Input: dimensioned drawing with shaded views. Units: mm. Origin: part minimum x, y, z. A direction names the side the tool comes from. Round coordinates to 2 decimals unless told otherwise and drop trailing zeros. Order: outer loops, then holes, each group sorted by start corner. A loop starts at its lowest first (then second) coordinate and runs counter-clockwise, first axis right, second up. Notation, with made-up numbers: (82.25, 55.25) - (89.25, 55.25) arc R24 cw to (89.25, 70.25) - close; hole circle Ø9 at (16.25, -10). An arc over 180 degrees is marked (long way). One line per item, written item: value. Start each with the question number.
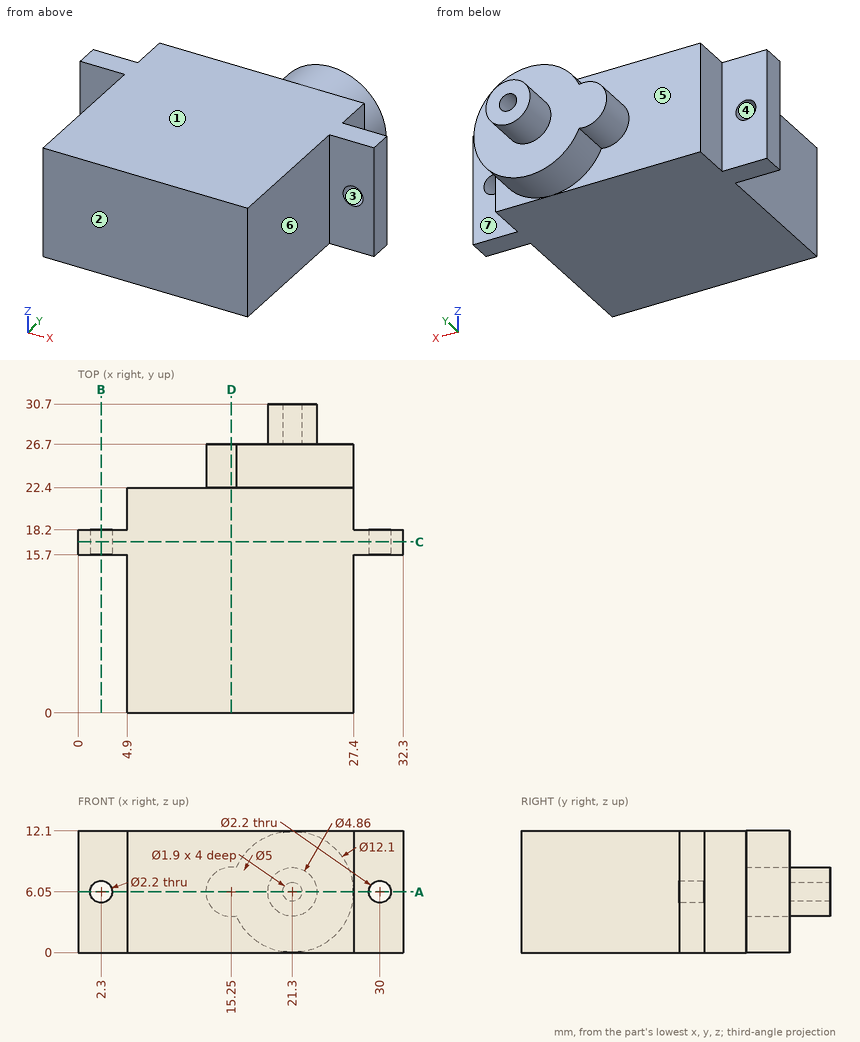
1. Set-up query: the marked faces 5, 6 and 7. Return all of +Z, -Z, +X, -X, +Y, -Y with unobstructed straight access to the full face (end or side cutting, diameter ignored); none if empty.
2. Section C-C (y = 17). Return the cut outline in (x, z).
3. Section A-A (z = 6.05). State how many separate pieces and enclosed holes the cut face has, then the cut area to 3 significant figures.
4. Section B-B (x = 2.3). Return the cut outline in (y, z), then the cut area to 4 significant figures.
5. Line query: line 1 (X direction, y = 16.7, z = 6.05); line 2 (X direction, y = 29.75, z = 6.05); line 3 (Z direction, x = 30, y = 17.2). Output: solid intervals per line, ascending. Write a range as from..to.
6. Pin query (flat end, axial travel): pin 1 (1.5 mm diameter, centred on x = 2.5, z = 7, fed in from -Y); pin 2 (8 mm diameter, centred on x = 18.5, y = 26, fed in from +Z); pin 3 (1.7 mm diameter, centred on x = 21.3, z = 6.05, fed in from +Y); pin 4 (6 mm diameter, centred on x = 11.5, y = 26, fed in from -Z). Return the tip coordinate at first contact, or that it passes through.
7. Section D-D (x = 15.25). Return the cut outline in (y, z), then the cut area to 3 significant figures.
8. Pull-direction query (Z, two-part tool) for the marked faces 1, 2, 3 and 4; classes: released by +Z, released by -Z, zero draft, split by the parting line, or undercut.
Solved:
1. face 5: -X, +Y
1. face 6: +Z, -Z, +X, -Y
1. face 7: +Z, -Z, +X, +Y
2. outline: (0, 0) - (32.3, 0) - (32.3, 12.1) - (0, 12.1) - close; hole circle Ø2.2 at (2.3, 6.05); hole circle Ø2.2 at (30, 6.05)
3. separate pieces: 3
3. enclosed holes: 0
3. area: 592 mm²
4. outline: (15.7, 0) - (18.2, 0) - (18.2, 4.95) - (15.7, 4.95) - close; (15.7, 7.15) - (18.2, 7.15) - (18.2, 12.1) - (15.7, 12.1) - close
4. area: 24.75 mm²
5. line 1: x = 0..1.2, 3.4..28.9, 31.1..32.3
5. line 2: x = 18.87..20.35, 22.25..23.73
5. line 3: z = 0..4.95, 7.15..12.1
6. pin 1: stops at y = 15.7
6. pin 2: stops at z = 12.1
6. pin 3: stops at y = 26.7
6. pin 4: stops at z = 3.67
7. outline: (0, 0) - (22.4, 0) - (22.4, 3.55) - (26.7, 3.55) - (26.7, 8.55) - (22.4, 8.55) - (22.4, 12.1) - (0, 12.1) - close
7. area: 293 mm²
8. face 1: released by +Z
8. face 2: zero draft
8. face 3: undercut
8. face 4: undercut
